Geometry check sheet. Reference: the model listing, model coordinates, mm. Face numbers are marked on the shaded views. A direction names the side the tool comes from. Round coordinates to 2 decimals unless told otherwise and drop trailing zeros. Order: outer loops, then holes, each group sorted by start corner. A loop starts at its lowest first (then second) coordinate and runs counter-clockwise, first axis right, second up.
(1) Set-up check for the marked faces 4 and 5: record each of +Z, -Z, +X, -X, +Y, -Y from which the full face is reachable in a straight line by a thin tool's end or side.
(2) Go/stop test with flat-tipped pins: pin 1 (4.5 mm diameter, centred on x = -11.67, y = 2.78, fed in from +Z); pin 2 (2 mm diameter, centred on x = 7.5, z = 4, fed in from +Y); pin 3 (1 mm diameter, centred on x = -19, z = 2.5, fed in from +Y). Record where each tip stops, or that it passes through.
(3) Sectioned sample at B-B (z = 5.75). Record the boundary of the cut face in (x, y), plus the area to 3 significant figures.
(4) Material ranges on line 1 along X through (y, z) = (2.5, 4.25); line 2 along Y through (x, z) = (0, 4.25); line 3 along Y through (x, z) = (-1, 5.25), recorded low to high.
(5) Release check for a two-part mould opening along Y. For the marked faces 1, 2 and 3 record: +Y half, -Y half, draft (parallel to the pull), parting line (faces both ways), or undercut.
(6) Sectioned sample at D-D (z = 2.5). Record the boundary of the cut face in (x, y).
(7) Sectioned sample at C-C (y = -6). Record the boundary of the cut face in (x, z), plus the area to 3 significant figures.
(8) Sectioned sample at A-A (x = 8). Record the boundary of the cut face in (y, z).
from build123d import *

# Parameters (mm, degrees)
F0_R     = 25.4
F0_R_2   = 6.35
F1_DEPTH = 7.112
F2_R     = 2.921
F3_DEPTH = 25.4
F4_R     = 3.181952
F4_R_2   = 1.778
F4_R_3   = 3.147606
F4_R_4   = 3.161985
F4_R_5   = 3.109144
F5_DEPTH = 3.302


with BuildPart() as f1:
    # F0 (on Top) → F1 (new body)
    with BuildSketch(Plane.XY):
        with Locations((-1.887769, 2.777323)):
            Circle(F0_R)
        with Locations((-1.887769, 2.777323)):
            Circle(F0_R_2, mode=Mode.SUBTRACT)
    extrude(amount=F1_DEPTH)

    # F2 (on face) → F3 (cut)
    with BuildSketch(Plane.XY.offset(7.112)):
        with BuildLine():
            ThreePointArc((1.033231, 12.556323), (-3.953228, 14.621782), (-1.887769, 9.635323))
            ThreePointArc((-1.887769, 9.635323), (0.17769, 10.490864), (1.033231, 12.556323))
        make_face()
        with BuildLine():
            ThreePointArc((1.033231, -7.001677), (0.17769, -4.936218), (-1.887769, -4.080677))
            ThreePointArc((-1.887769, -4.080677), (-3.953228, -9.067136), (1.033231, -7.001677))
        make_face()
        with Locations((-11.666769, 2.777323)):
            Circle(F2_R)
        with BuildLine():
            ThreePointArc((10.812231, 2.777323), (7.891231, 5.698323), (4.970231, 2.777323))
            ThreePointArc((4.970231, 2.777323), (7.891231, -0.143677), (10.812231, 2.777323))
        make_face()
    extrude(amount=-F3_DEPTH, mode=Mode.SUBTRACT)

    # F4 (on face) → F5 (join)
    with BuildSketch(Plane(origin=(0, 0, 0), x_dir=(1, 0, 0), z_dir=(0, 0, -1))):
        with Locations((-1.887769, 7.001677)):
            Circle(F4_R)
        with Locations((-1.887769, 7.001677)):
            Circle(F4_R_2, mode=Mode.SUBTRACT)
        with Locations((7.891231, -2.777323)):
            Circle(F4_R_3)
        with Locations((7.891231, -2.777323)):
            Circle(F4_R_2, mode=Mode.SUBTRACT)
        with Locations((-1.887769, -12.556323)):
            Circle(F4_R_4)
        with Locations((-1.887769, -12.556323)):
            Circle(F4_R_2, mode=Mode.SUBTRACT)
        with Locations((-11.666769, -2.777323)):
            Circle(F4_R_5)
        with Locations((-11.666769, -2.777323)):
            Circle(F4_R_2, mode=Mode.SUBTRACT)
    extrude(amount=-F5_DEPTH)


solid = f1.part
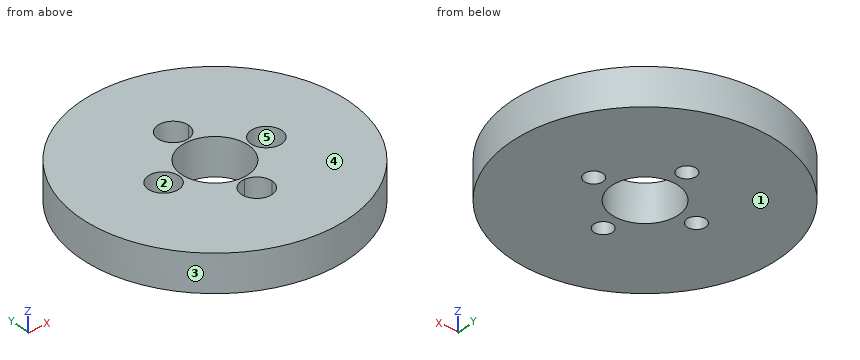
Answer below:
1. face 4: +Z, +X, -X, +Y, -Y
1. face 5: +Z
2. pin 1: stops at z = 3.3
2. pin 2: stops at y = 26.75
2. pin 3: stops at y = 21.99
3. outline: circle Ø50.8 at (-1.89, 2.78); hole circle Ø5.84 at (-11.67, 2.78); hole circle Ø12.7 at (-1.89, 2.78); hole circle Ø5.84 at (-1.89, -7); hole circle Ø5.84 at (-1.89, 12.56); hole circle Ø5.84 at (7.89, 2.78)
3. area: 1,790 mm2
4. line 1: x = -27.29 to -14.57, -8.76 to -8.23, 4.46 to 4.98, 10.8 to 23.51
4. line 2: y = -22.55 to -9.23, -4.77 to -3.29, 8.84 to 10.33, 14.79 to 28.11
4. line 3: y = -22.61 to -9.78, -4.22 to -3.51, 9.06 to 9.77, 15.34 to 28.16
5. face 1: draft
5. face 2: undercut
5. face 3: parting line
6. outline: circle Ø50.8 at (-1.89, 2.78); hole circle Ø3.56 at (-11.67, 2.78); hole circle Ø12.7 at (-1.89, 2.78); hole circle Ø3.56 at (-1.89, -7); hole circle Ø3.56 at (-1.89, 12.56); hole circle Ø3.56 at (7.89, 2.78)
7. outline: (-25.72, 0) - (-3.36, 0) - (-3.36, 3.3) - (-4.63, 3.3) - (-4.63, 7.11) - (-25.72, 7.11) - close; (-0.42, 0) - (21.95, 0) - (21.95, 7.11) - (0.86, 7.11) - (0.86, 3.3) - (-0.42, 3.3) - close
7. area: 308 mm2
8. outline: (-20.62, 0) - (1, 0) - (1, 3.3) - (-0.14, 3.3) - (-0.14, 7.11) - (-20.62, 7.11) - close; (4.55, 0) - (26.17, 0) - (26.17, 7.11) - (5.7, 7.11) - (5.7, 3.3) - (4.55, 3.3) - close
